Geometry check sheet. Reference: the model listing, model coordinates, mm. Face numbers are marked on the shaded views. Coordinates: 2 decimals unless noted, no trailing zeros. Order: outer loops, then holes, each group sorted by start corner. A loop starts at its lowest first (then second) coordinate and runs counter-clockwise, first axis right, second up. Notation, with made-up numbers: (-34, 79.5) - (-12, 79.5) arc R36 cw to (-12, 117.5) - close; hole circle Ø9 at (64.5, -25). An arc over 180 degrees is marked (long way). Use CSV: the item, a comma, the result in double quotes. Start each with the question number.
1) Sectioned sample at A-A, the plane x = 0. Record the cut outline in (y, z).
2) Sectioned sample at B-B, the plane y = -5.5. Record the cut outline in (x, z), and give its area (3 significant figures).
3) Draft check along X on the marked faces 1, 2, 3 and 4. Enter one of: released by +X, released by -X, zero draft, split by the parting line, or undercut.
4) Thickness scan on probe 1 along Y at (x, z) = (7.5, 4.75); probe 2 along Y at (x, z) = (0.25, 0); probe 3 along Y at (x, z) = (-7, -3). Record the ranges inside material, lowest first. Write a range as [from, to].
from build123d import *

# Parameters (mm, degrees)
SKETCH1_W           = 20.917422255
SKETCH1_H           = 21.921735574
BOSS_EXTRUDE1_DEPTH = 5


with BuildPart() as part:
    # Sketch1 → Boss-Extrude1 (new body, symmetric)
    with BuildSketch(Plane.XY):
        with Locations((0.415577926, 1.038944814)):
            Rectangle(SKETCH1_W, SKETCH1_H)
        with BuildLine():
            Line((-1, 6.422616289), (-1, 7.422616289))
            Line((-1, 7.422616289), (-0.5, 8.622616289))
            Line((-0.5, 8.622616289), (0.5, 8.622616289))
            Line((0.5, 8.622616289), (1, 7.422616289))
            Line((1, 7.422616289), (1, 6.422616289))
            ThreePointArc((1, 6.422616289), (1.682323793, 6.278517871), (2.345282741, 6.062148865))
            Line((2.345282741, 6.062148865), (2.845282741, 6.928174269))
            Line((2.845282741, 6.928174269), (3.878295443, 7.717404754))
            Line((3.878295443, 7.717404754), (4.744320847, 7.217404754))
            Line((4.744320847, 7.217404754), (4.577333548, 5.928174269))
            Line((4.577333548, 5.928174269), (4.077333548, 5.062148865))
            ThreePointArc((4.077333548, 5.062148865), (4.596194078, 4.596194078), (5.062148865, 4.077333548))
            Line((5.062148865, 4.077333548), (5.928174269, 4.577333548))
            Line((5.928174269, 4.577333548), (7.217404754, 4.744320847))
            Line((7.217404754, 4.744320847), (7.717404754, 3.878295443))
            Line((7.717404754, 3.878295443), (6.928174269, 2.845282741))
            Line((6.928174269, 2.845282741), (6.062148865, 2.345282741))
            ThreePointArc((6.062148865, 2.345282741), (6.278517871, 1.682323793), (6.422616289, 1))
            Line((6.422616289, 1), (7.422616289, 1))
            Line((7.422616289, 1), (8.622616289, 0.5))
            Line((8.622616289, 0.5), (8.622616289, -0.5))
            Line((8.622616289, -0.5), (7.422616289, -1))
            Line((7.422616289, -1), (6.422616289, -1))
            ThreePointArc((6.422616289, -1), (6.278517871, -1.682323793), (6.062148865, -2.345282741))
            Line((6.062148865, -2.345282741), (6.928174269, -2.845282741))
            Line((6.928174269, -2.845282741), (7.717404754, -3.878295443))
            Line((7.717404754, -3.878295443), (7.217404754, -4.744320847))
            Line((7.217404754, -4.744320847), (5.928174269, -4.577333548))
            Line((5.928174269, -4.577333548), (5.062148865, -4.077333548))
            ThreePointArc((5.062148865, -4.077333548), (4.596194078, -4.596194078), (4.077333548, -5.062148865))
            Line((4.077333548, -5.062148865), (4.577333548, -5.928174269))
            Line((4.577333548, -5.928174269), (4.744320847, -7.217404754))
            Line((4.744320847, -7.217404754), (3.878295443, -7.717404754))
            Line((3.878295443, -7.717404754), (2.845282741, -6.928174269))
            Line((2.845282741, -6.928174269), (2.345282741, -6.062148865))
            ThreePointArc((2.345282741, -6.062148865), (1.682323793, -6.278517871), (1, -6.422616289))
            Line((1, -6.422616289), (1, -7.422616289))
            Line((1, -7.422616289), (0.5, -8.622616289))
            Line((0.5, -8.622616289), (-0.5, -8.622616289))
            Line((-0.5, -8.622616289), (-1, -7.422616289))
            Line((-1, -7.422616289), (-1, -6.422616289))
            ThreePointArc((-1, -6.422616289), (-1.682323793, -6.278517871), (-2.345282741, -6.062148865))
            Line((-2.345282741, -6.062148865), (-2.845282741, -6.928174269))
            Line((-2.845282741, -6.928174269), (-3.878295443, -7.717404754))
            Line((-3.878295443, -7.717404754), (-4.744320847, -7.217404754))
            Line((-4.744320847, -7.217404754), (-4.577333548, -5.928174269))
            Line((-4.577333548, -5.928174269), (-4.077333548, -5.062148865))
            ThreePointArc((-4.077333548, -5.062148865), (-4.596194078, -4.596194078), (-5.062148865, -4.077333548))
            Line((-5.062148865, -4.077333548), (-5.928174269, -4.577333548))
            Line((-5.928174269, -4.577333548), (-7.217404754, -4.744320847))
            Line((-7.217404754, -4.744320847), (-7.717404754, -3.878295443))
            Line((-7.717404754, -3.878295443), (-6.928174269, -2.845282741))
            Line((-6.928174269, -2.845282741), (-6.062148865, -2.345282741))
            ThreePointArc((-6.062148865, -2.345282741), (-6.278517871, -1.682323793), (-6.422616289, -1))
            Line((-6.422616289, -1), (-7.422616289, -1))
            Line((-7.422616289, -1), (-8.622616289, -0.5))
            Line((-8.622616289, -0.5), (-8.622616289, 0.5))
            Line((-8.622616289, 0.5), (-7.422616289, 1))
            Line((-7.422616289, 1), (-6.422616289, 1))
            ThreePointArc((-6.422616289, 1), (-6.278517871, 1.682323793), (-6.062148865, 2.345282741))
            Line((-6.062148865, 2.345282741), (-6.928174269, 2.845282741))
            Line((-6.928174269, 2.845282741), (-7.717404754, 3.878295443))
            Line((-7.717404754, 3.878295443), (-7.217404754, 4.744320847))
            Line((-7.217404754, 4.744320847), (-5.928174269, 4.577333548))
            Line((-5.928174269, 4.577333548), (-5.062148865, 4.077333548))
            ThreePointArc((-5.062148865, 4.077333548), (-4.596194078, 4.596194078), (-4.077333548, 5.062148865))
            Line((-4.077333548, 5.062148865), (-4.577333548, 5.928174269))
            Line((-4.577333548, 5.928174269), (-4.744320847, 7.217404754))
            Line((-4.744320847, 7.217404754), (-3.878295443, 7.717404754))
            Line((-3.878295443, 7.717404754), (-2.845282741, 6.928174269))
            Line((-2.845282741, 6.928174269), (-2.345282741, 6.062148865))
            ThreePointArc((-2.345282741, 6.062148865), (-1.682323793, 6.278517871), (-1, 6.422616289))
        make_face(mode=Mode.SUBTRACT)
    extrude(amount=BOSS_EXTRUDE1_DEPTH, both=True)


solid = part.part
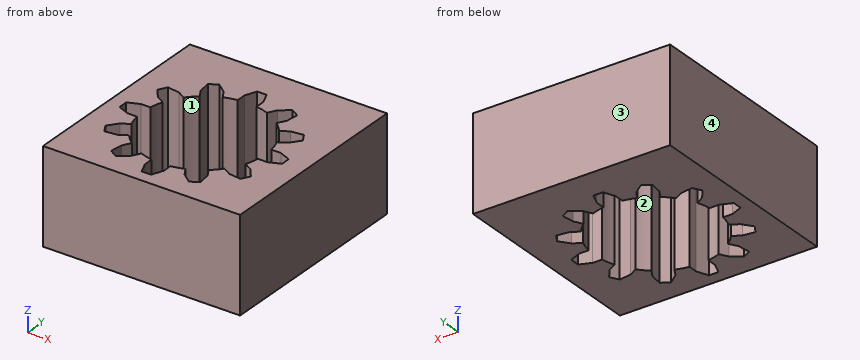
Evaluation:
1,outline,"(-9.92, -5) - (-8.62, -5) - (-8.62, 5) - (-9.92, 5) - close; (8.62, -5) - (12, -5) - (12, 5) - (8.62, 5) - close"
2,outline,"(-10.04, -5) - (-4.33, -5) - (-4.33, 5) - (-10.04, 5) - close; (4.33, -5) - (10.87, -5) - (10.87, 5) - (4.33, 5) - close"
2,area,"123 mm²"
3,face 1,"undercut"
3,face 2,"undercut"
3,face 3,"zero draft"
3,face 4,"released by -X"
4,probe 1,"[-9.92, -4.25], [-3.59, -0.97], [0.97, 3.59], [4.25, 12]"
4,probe 2,"[-9.92, -8.62], [8.62, 12]"
4,probe 3,"[-9.92, -4.72], [-2.94, -1], [1, 2.94], [4.72, 12]"
